from build123d import *

# Parameters (mm, degrees)
F1_DEPTH = 3
F2_R     = 2.5
F3_DEPTH = 3
F4_R     = 3
F5_DEPTH = 3
F6_R     = 2.1
F7_DEPTH = 3
F8_W     = 20
F8_H     = 3
F9_DEPTH = 3
F10_R    = 4.99999


# Not quite as in the source:
# - a fillet or chamfer is up to 0.001 mm smaller than in the source, because OpenCascade refuses the exact size


with BuildPart() as f1:
    # F0 (on Front) → F1 (new body)
    with BuildSketch(Plane.XZ):
        Polygon((140, -105), (145, -105), (145, 105), (-145, 105), (-145, -105), (-140, -105), (-140, -95), (-134.5, -95), (-134.5, -105), (134.5, -105), (134.5, -95), (140, -95), align=None)
    extrude(amount=F1_DEPTH)

    # F2 (on face) → F3 (cut, through all)
    with BuildSketch(Plane.XZ.offset(3)):
        with Locations((-70, 100)):
            Circle(F2_R)
        with Locations((-70, 30)):
            Circle(F2_R)
        with Locations((70, 100)):
            Circle(F2_R)
        with Locations((70, 30)):
            Circle(F2_R)
    extrude(amount=-F3_DEPTH, mode=Mode.SUBTRACT)

    # F4 (on face) → F5 (cut, through all)
    with BuildSketch(Plane.XZ.offset(3)):
        with Locations((102.5, -30)):
            Circle(F4_R)
        with Locations((-102.5, -30)):
            Circle(F4_R)
    extrude(amount=-F5_DEPTH, mode=Mode.SUBTRACT)

    # F6 (on face) → F7 (cut, through all)
    with BuildSketch(Plane.XZ.offset(3)):
        with Locations((118, 65)):
            Circle(F6_R)
        with Locations((140, 65)):
            Circle(F6_R)
    extrude(amount=-F7_DEPTH, mode=Mode.SUBTRACT)

    # F8 (on face) → F9 (cut, through all)
    with BuildSketch(Plane.XZ.offset(3)):
        with Locations((-55, -85)):
            Rectangle(F8_W, F8_H)
        with Locations((45, -85)):
            Rectangle(F8_W, F8_H)
        with Locations((45, -100)):
            Rectangle(F8_W, F8_H)
        with Locations((-55, -100)):
            Rectangle(F8_W, F8_H)
    extrude(amount=-F9_DEPTH, mode=Mode.SUBTRACT)

    # F10 (radius 5 in the source; OpenCascade refuses exactly that, so slightly less here)
    f10_edges = [f1.edges().sort_by_distance(p)[0] for p in [
        (-145, -1.5, 105),
        (-145, -1.5, -105),
        (145, -1.5, -105),
        (145, -1.5, 105),
    ]]
    fillet(f10_edges, radius=F10_R)


solid = f1.part
Source: CAD feature listing. Evaluate the final solid. Frame: model axes, mm. Coordinates: 2 decimals unless noted, no trailing zeros. Loops run counter-clockwise (first coordinate to the right, second up) from the corner with the lowest first, then second, coordinate; pieces in that order, holes last. Notation, with made-up numbers: (10, 59.25) - (57, 59.25) arc R13 ccw to (57, 70.25) - close; hole circle Ø3 at (47, 27.25). An arc over 180 degrees is marked (long way). One line per question, with ' | ' between items.
1) Section A-A, the plane x = 102.5. Return loops of the section in (y, z), then the cut area to 3 significant figures.
Report:
outline: (-3, -105) - (0, -105) - (0, -33) - (-3, -33) - close; (-3, -27) - (0, -27) - (0, 105) - (-3, 105) - close | area: 612 mm²
2) Line query: line 1 along Z through (x, y) = (-70, -2.25); line 2 along Z through (x, y) = (-62, -2.45); line 3 along X through (y, z) = (-1.1, 64.5). Output: solid intervals per line, ascending.
Report:
line 1: z = -105 to 27.5, 32.5 to 97.5, 102.5 to 105 | line 2: z = -105 to -101.5, -98.5 to -86.5, -83.5 to 105 | line 3: x = -145 to 115.96, 120.04 to 137.96, 142.04 to 145
3) Pull-direction query (X, two-part tool) for faces 1 (the face through (100.1, -1.5, -31.8)), 2 (the face through (-2, -3, 1)); classes: released by +X, released by -X, zero draft, split by the parting line, or undercut.
Report:
face 1: undercut | face 2: zero draft
4) First-contact query: P1, Ø1.5, axis at x = 137.5, y = -1.5, coming from the -Z side; P2, Ø1.5, axis at y = -1, z = -102, coming from the -X side. Flat tips, straight axial feed; report the tip coordinate or a pass-through.
Report:
P1: stops at z = -95 | P2: stops at x = -144.84
